Job drawing, mm, ordinate dimensions from the low corner. One solid piece. A direction names the side the tool comes from. Coordinates: 2 decimals unless noted, no trailing zeros. Write each loop counter-clockwise with the first axis right and the second up, starting at its lowest first coordinate (ties: lowest second). Pieces come first, ordered by that corner, then holes. Notation, with made-up numbers: (-22, -8.5) - (18, -8.5) arc R20 ccw to (18, 0.5) - close; hole circle Ø9 at (-1, 32). An arc over 180 degrees is marked (long way). Use one line per item in the form item = value. Start each with the question number.
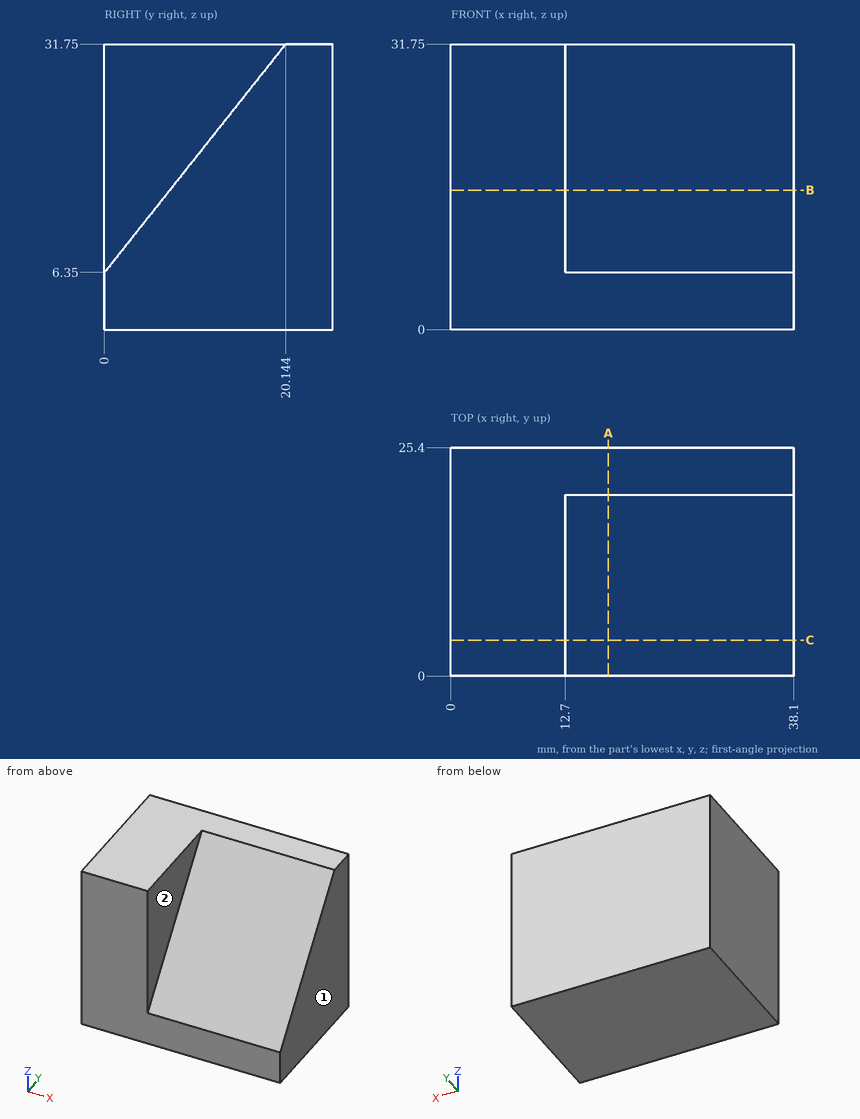
Q1. Slice it at A-A (x = 17.5). List the corners of the cut face in (y, z), plus the area to 3 significant figures.
Q2. Slice it at B-B (z = 15.5). List the corners of the cut face in (x, y), plus the area to 3 significant figures.
Q3. Which spindle directions (+Z, -Z, +X, -X, +Y, -Y) get a long thin tool onto all of the face, cutting with end or side? Do the marked faces 1 and 2. Say none if no direction does.
Q4. Drill centre lines: probe 1 along X at (y, z) = (10.75, 20); probe 2 along Y at (x, z) = (24.5, 18); probe 3 along Y at (x, z) = (36, 27). Where is each one in solid material? Low to high.
Q5. Slice it at C-C (y = 4). List the corners of the cut face in (x, z).
Solution:
q1.outline = (0, 0) - (25.4, 0) - (25.4, 31.75) - (20.14, 31.75) - (0, 6.35) - close
q1.area = 551 mm2
q2.outline = (0, 0) - (12.7, 0) - (12.7, 7.26) - (38.1, 7.26) - (38.1, 25.4) - (0, 25.4) - close
q2.area = 783 mm2
q3.face_1 = +Z, -Z, +X, +Y, -Y
q3.face_2 = +Z, +X, -Y
q4.probe_1 = 0 to 12.7
q4.probe_2 = 9.24 to 25.4
q4.probe_3 = 16.38 to 25.4
q5.outline = (0, 0) - (38.1, 0) - (38.1, 11.39) - (12.7, 11.39) - (12.7, 31.75) - (0, 31.75) - close
